Here's how the part is built. I have some questions about the finished solid (model axes, mm). Face numbers are marked on the shaded views. A direction names the side the tool comes from. Coordinates: 2 decimals unless noted, no trailing zeros. Write each loop counter-clockwise with the first axis right and the second up, starting at its lowest first coordinate (ties: lowest second). Pieces come first, ordered by that corner, then holes. Notation, with made-up numbers: (38.5, -28.75) -> (50.5, -28.75) arc R18 ccw to (50.5, -8.75) -> close; hole circle Ø1 at (52, 21). An arc over 180 degrees is marked (long way). Use a Markdown table: item, result. Add a question column.
Item 1: On a 3-axis mill with a long thin cutter (end or side, diameter ignored), from which of +Z, -Z, +X, -X, +Y, -Y can I reach the whole of each face in a straight line? I mean the marked faces 1, 2, 3, 4 and 5. Say none if no direction works.
Item 2: Imagine slicing it at B-B, the plane x = -1.5. Write out the boundary of the cut face in (y, z).
Item 3: Imagine slicing it at C-C, the plane x = 15. Write out the boundary of the cut face in (y, z).
Item 4: Imagine slicing it at A-A, the plane z = 2. Write out the boundary of the cut face in (x, y).
Item 5: Will these pins go through, and if not, where does the flat tip stop? pin 1 Ø3 at (x, z) = (18, 13) entering from -Y; pin 2 Ø11 at (y, z) = (20.5, 16.5) entering from -X; pin 3 Ø1 at (x, y) = (10, -19.5) entering from +Z; pin 4 Ø2 at (x, y) = (5, 2) entering from +Z.
Item 6: If I drill on line 1 along X through (y, z) = (17, 15.5); line 2 along Z through (x, y) = (2, -20), over which ranges is the centre line in solid material (lowest first)? Write a range as from..to.
Item 7: Imagine slicing it at D-D, the plane z = 17.25. Write out the boundary of the cut face in (x, y), and give its area (3 significant figures).
```python
from build123d import *

# Parameters (mm, degrees)
ESTRUSIONE_ESTRUSIONE1_DEPTH = 20
ESTRUSIONE_ESTRUSIONE3_DEPTH = 10
TAGLIO_ESTRUSIONE2_DEPTH     = 51.497524692
SMUSSO2_SIZE                 = 3
RACCORDO3_R                  = 20


with BuildPart() as part:
    # Schizzo1 → Estrusione-Estrusione1 (new body)
    with BuildSketch(Plane.XY):
        with BuildLine():
            Line((-15, 0), (0, -15))
            Line((0, -15), (30, -15))
            Line((30, -15), (30, 0))
            Line((30, 0), (2.5, 0))
            ThreePointArc((2.5, 0), (-1.767766953, -1.767766953), (0, 2.5))
            Line((0, 2.5), (0, 30))
            Line((0, 30), (-15, 30))
            Line((-15, 30), (-15, 0))
        make_face()
    extrude(amount=ESTRUSIONE_ESTRUSIONE1_DEPTH)

    # Schizzo2 → Estrusione-Estrusione3 (add)
    with BuildSketch(Plane(origin=(0, 0, 0), x_dir=(-1, 0, 0), z_dir=(0, 0, -1))):
        Polygon((35, 0), (15, 30), (15, 0), (0, -15), (-30, -15), (0, -35), align=None)
    extrude(amount=-ESTRUSIONE_ESTRUSIONE3_DEPTH)

    # Schizzo4 → Taglio-Estrusione2 (cut, through all)
    with BuildSketch(Plane.XY.offset(10)):
        with BuildLine():
            ThreePointArc((-9.5, -12.5), (-9.728361402, -11.351949703), (-10.378679656, -10.378679656))
            Line((-10.378679656, -10.378679656), (-14.621320344, -14.621320344))
            ThreePointArc((-14.621320344, -14.621320344), (-11.351949703, -15.271638598), (-9.5, -12.5))
        make_face()
        with BuildLine():
            Line((-14.621320344, -14.621320344), (-10.378679656, -10.378679656))
            ThreePointArc((-10.378679656, -10.378679656), (-14.621320344, -10.378679656), (-14.621320344, -14.621320344))
        make_face()
    extrude(amount=-TAGLIO_ESTRUSIONE2_DEPTH, mode=Mode.SUBTRACT)

    # Smusso2
    smusso2_edges = [part.edges().sort_by_distance(p)[0] for p in [
        (-10.378679656, -10.378679656, 10),
    ]]
    chamfer(smusso2_edges, length=SMUSSO2_SIZE)

    # Raccordo3
    raccordo3_edges = [part.edges().sort_by_distance(p)[0] for p in [
        (0, -15, 15),
        (-15, 0, 15),
        (-35, 0, 5),
        (0, -35, 5),
    ]]
    fillet(raccordo3_edges, radius=RACCORDO3_R)


solid = part.part
```
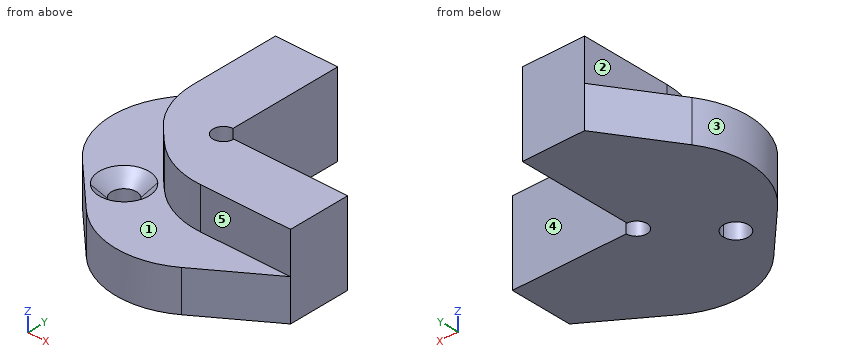
Ans:
| question | item | result |
|---|---|---|
| 1 | face 1 | +Z, -X, -Y |
| 1 | face 2 | +Z, -X, +Y, -Y |
| 1 | face 3 | +Z, -Z, -X |
| 1 | face 4 | +Z, -Z, +X, +Y |
| 1 | face 5 | +Z, +X, -X, -Y |
| 2 | outline | (-28.85, 0) -> (-2, 0) -> (-2, 20) -> (-12.44, 20) -> (-12.44, 10) -> (-28.85, 10) -> close; (2, 0) -> (30, 0) -> (30, 20) -> (2, 20) -> close |
| 3 | outline | (-25, 0) -> (0, 0) -> (0, 20) -> (-15, 20) -> (-15, 10) -> (-25, 10) -> close |
| 4 | outline | (-25.91, 13.64) arc R20 ccw to (-23.41, -11.59) -> (-11.59, -23.41) arc R20 ccw to (13.64, -25.91) -> (30, -15) -> (30, 0) -> (2.5, 0) arc R2.5 cw (long way) to (0, 2.5) -> (0, 30) -> (-15, 30) -> close; hole circle Ø6 at (-12.5, -12.5) |
| 5 | pin 1 | stops at y = -15 |
| 5 | pin 2 | stops at x = -15 |
| 5 | pin 3 | stops at z = 10 |
| 5 | pin 4 | passes through |
| 6 | line 1 | x = -15..0 |
| 6 | line 2 | z = 0..10 |
| 7 | outline | (-15, 8.28) arc R20 ccw to (-9.14, -5.86) -> (-5.86, -9.14) arc R20 ccw to (8.28, -15) -> (30, -15) -> (30, 0) -> (2.5, 0) arc R2.5 cw (long way) to (0, 2.5) -> (0, 30) -> (-15, 30) -> close |
| 7 | area | 981 mm^2 |
